Part print with two shaded views. Sizes in mm from the minimum x, y, z corner. A direction names the side the tool comes from. Coordinates: 2 decimals unless noted, no trailing zeros. Loops run counter-clockwise (first coordinate to the right, second up) from the corner with the lowest first, then second, coordinate; pieces in that order, holes last.
(1) Slice it at D-D (y = 521.5). Give the cut face in (x, z), and give its area (3 significant figures).
(2) Slice it at B-B (y = 151). Give the cut face in (x, z).
(3) Slice it at C-C (x = 635). Give the cut face in (y, z).
(4) Flat gauge pins, fed straight in: P1, Ø6, axis at x = 257, z = 194, coming from the +Y side (1 decimal); P2, Ø3, axis at x = 533.5, z = 586.5, coming from the +Y side; P3, Ø4, axis at x = 206, z = 716.5, coming from the -Y side; P4, Ø3, axis at y = 1270, z = 704.5, coming from the +X side. Where does each tip first touch, or does it go through?
(5) Wall check: L1, parallel to Y at x = 884, z = 359.5; L2, parallel to Z at x = 1270, y = 439. Give the ranges that are in metal, low to high.
(6) Tool access for the marked faces 1, 2 and 3: list every direction of +Z, -Z, +X, -X, +Y, -Y with a clear straight run to the whole face (end or side of a thin tool).
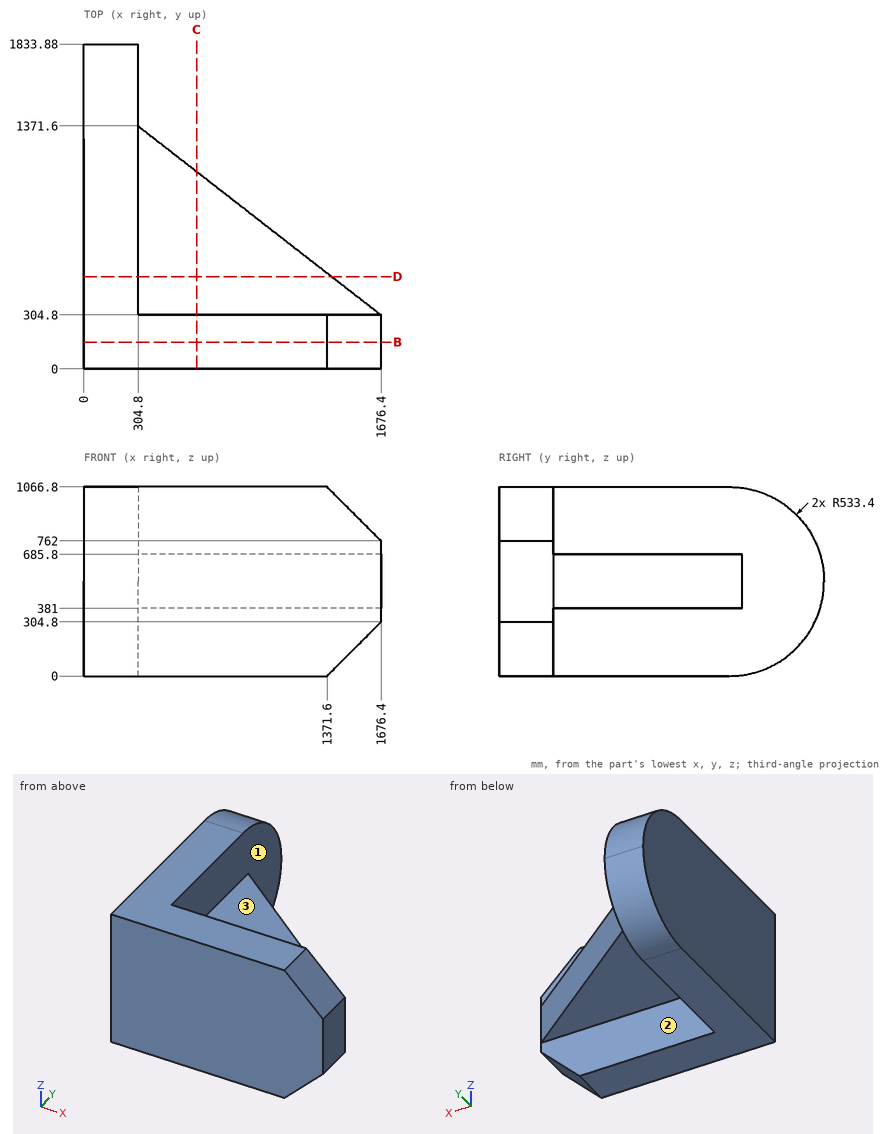
Response values:
1. outline: (0, 0) - (304.8, 0) - (304.8, 381) - (1397.79, 381) - (1397.79, 685.8) - (304.8, 685.8) - (304.8, 1066.8) - (0, 1066.8) - close
1. area: 658,000 mm2
2. outline: (0, 0) - (1371.6, 0) - (1676.4, 304.8) - (1676.4, 762) - (1371.6, 1066.8) - (0, 1066.8) - close
3. outline: (0, 0) - (304.8, 0) - (304.8, 381) - (1114.78, 381) - (1114.78, 685.8) - (304.8, 685.8) - (304.8, 1066.8) - (0, 1066.8) - close
4. P1: stops at y = 1714.4
4. P2: stops at y = 1194.89
4. P3: stops at y = 0
4. P4: stops at x = 304.8
5. L1: y = 0 to 304.8
5. L2: z = 381 to 685.8
6. face 1: +X, +Y
6. face 2: -Z, +X, +Y
6. face 3: +Z, +X, +Y
